```python
from build123d import *

# Parameters (mm, degrees)
SKETCH_W        = 30
SKETCH_H        = 200
PAD_DEPTH       = 10
POCKET_DEPTH    = 7.1
SKETCH002_W     = 200
SKETCH002_H     = 4.1
POCKET001_DEPTH = 7.1
SKETCH003_R     = 1.6
POCKET002_DEPTH = 25
SKETCH004_W     = 2.6
SKETCH004_H     = 5.7
POCKET003_DEPTH = 6.15
SKETCH006_W     = 200
SKETCH006_H     = 3
POCKET005_DEPTH = 5.9
POCKET006_DEPTH = 10
SKETCH008_W     = 5.9
SKETCH008_H     = 200
POCKET007_DEPTH = 3
POCKET008_DEPTH = 5.1
SKETCH010_W     = 30
SKETCH010_H     = 6.1
POCKET009_DEPTH = 5.1
POCKET010_DEPTH = 5


with BuildPart() as part:
    # Sketch → Pad (new body)
    with BuildSketch(Plane.XY):
        with Locations((15, 100)):
            Rectangle(SKETCH_W, SKETCH_H)
    extrude(amount=PAD_DEPTH)

    # Sketch001 (on Face4 of Pad) → Pocket (cut)
    with BuildSketch(Plane(origin=(0, 0, 0), x_dir=(0, -1, 0), z_dir=(-1, 0, 0))):
        Polygon((-199.7, 5.9), (-199.9, 0), (-179.9, 0), (-182.4, 5.9), align=None)
        Polygon((-167.6, 5.9), (-170.1, 0), (-154.9, 0), (-157.4, 5.9), align=None)
        Polygon((-142.6, 5.9), (-145.1, 0), (-129.9, 0), (-132.4, 5.9), align=None)
        Polygon((-117.6, 5.9), (-120.1, 0), (-104.9, 0), (-107.4, 5.9), align=None)
        Polygon((-92.6, 5.9), (-95.1, 0), (-79.9, 0), (-82.4, 5.9), align=None)
        Polygon((-67.6, 5.9), (-70.1, 0), (-54.9, 0), (-57.4, 5.9), align=None)
        Polygon((-42.6, 5.9), (-45.1, 0), (-29.9, 0), (-32.4, 5.9), align=None)
        Polygon((-17.6, 5.9), (-20.1, 0), (-4.9, 0), (-7.4, 5.9), align=None)
    extrude(amount=-POCKET_DEPTH, mode=Mode.SUBTRACT)

    # Sketch002 (on Face2 of Pocket) → Pocket001 (cut)
    with BuildSketch(Plane(origin=(0, 0, 0), x_dir=(0, -1, 0), z_dir=(-1, 0, 0))):
        with Locations((-100, 7.95)):
            Rectangle(SKETCH002_W, SKETCH002_H)
    extrude(amount=-POCKET001_DEPTH, mode=Mode.SUBTRACT)

    # Sketch003 (on Face9 of Pocket001) → Pocket002 (cut)
    with BuildSketch(Plane(origin=(7.1, 0, 0), x_dir=(0, -1, 0), z_dir=(-1, 0, 0))):
        with Locations((-37.5, 3)):
            Circle(SKETCH003_R)
        with Locations((-12.5, 3)):
            Circle(SKETCH003_R)
        with Locations((-62.5, 3)):
            Circle(SKETCH003_R)
        with Locations((-87.5, 3)):
            Circle(SKETCH003_R)
        with Locations((-112.5, 3)):
            Circle(SKETCH003_R)
        with Locations((-137.5, 3)):
            Circle(SKETCH003_R)
        with Locations((-162.5, 3)):
            Circle(SKETCH003_R)
        with Locations((-187.5, 3)):
            Circle(SKETCH003_R)
    extrude(amount=-POCKET002_DEPTH, mode=Mode.SUBTRACT)

    # Sketch004 (on Face2 of Pocket002) → Pocket003 (cut)
    with BuildSketch(Plane(origin=(0, 0, 0), x_dir=(1, 0, 0), z_dir=(0, 0, -1))):
        with Locations((15, -12.5)):
            Rectangle(SKETCH004_W, SKETCH004_H)
        with Locations((15, -37.5)):
            Rectangle(SKETCH004_W, SKETCH004_H)
        with Locations((15, -62.5)):
            Rectangle(SKETCH004_W, SKETCH004_H)
        with Locations((15, -87.5)):
            Rectangle(SKETCH004_W, SKETCH004_H)
        with Locations((15, -112.5)):
            Rectangle(SKETCH004_W, SKETCH004_H)
        with Locations((15, -137.5)):
            Rectangle(SKETCH004_W, SKETCH004_H)
        with Locations((15, -162.5)):
            Rectangle(SKETCH004_W, SKETCH004_H)
        with Locations((15, -187.5)):
            Rectangle(SKETCH004_W, SKETCH004_H)
    extrude(amount=-POCKET003_DEPTH, mode=Mode.SUBTRACT)

    # Sketch006 → Pocket005 (cut)
    with BuildSketch(Plane(origin=(0, 4.15414, -1.760229), x_dir=(-1, 0, 0), z_dir=(0, 0.920752, -0.390149))):
        with Locations((100, 8.5)):
            Rectangle(SKETCH006_W, SKETCH006_H)
    extrude(amount=-POCKET005_DEPTH, mode=Mode.SUBTRACT)

    # Sketch007 (on Face4 of Pocket005) → Pocket006 (cut)
    with BuildSketch(Plane.XY.offset(10)):
        Polygon((24.1, 20.1), (24.1, 4.9), (30, 7.4), (30, 17.6), align=None)
        Polygon((24.1, 45.1), (24.1, 29.9), (30, 32.4), (30, 42.6), align=None)
        Polygon((24.1, 70.1), (24.1, 54.9), (30, 57.4), (30, 67.6), align=None)
        Polygon((24.1, 95.1), (24.1, 79.9), (30, 82.4), (30, 92.6), align=None)
        Polygon((24.1, 120.1), (24.1, 104.9), (30, 107.4), (30, 117.6), align=None)
        Polygon((24.1, 145.1), (24.1, 129.9), (30, 132.4), (30, 142.6), align=None)
        Polygon((24.1, 170.1), (24.1, 154.9), (30, 157.4), (30, 167.6), align=None)
        Polygon((24.1, 195.1), (24.1, 179.9), (30, 182.4), (30, 192.6), align=None)
    extrude(amount=-POCKET006_DEPTH, mode=Mode.SUBTRACT)

    # Sketch008 (on Face4 of Pocket006) → Pocket007 (cut)
    with BuildSketch(Plane.XY.offset(10)):
        with Locations((27.05, 100)):
            Rectangle(SKETCH008_W, SKETCH008_H)
    extrude(amount=-POCKET007_DEPTH, mode=Mode.SUBTRACT)

    # Sketch009 (on Face6 of Pocket007) → Pocket008 (cut)
    with BuildSketch(Plane.XY.offset(10)):
        Polygon((7.4, 6.1), (22.6, 6.1), (20.1, 0), (9.9, 0), align=None)
    extrude(amount=-POCKET008_DEPTH, mode=Mode.SUBTRACT)

    # Sketch010 (on Face2 of Pocket008) → Pocket009 (cut)
    with BuildSketch(Plane(origin=(0, 0, 0), x_dir=(1, 0, 0), z_dir=(0, 0, -1))):
        with Locations((15, -196.95)):
            Rectangle(SKETCH010_W, SKETCH010_H)
    extrude(amount=-POCKET009_DEPTH, mode=Mode.SUBTRACT)

    # Sketch011 (on Face6 of Pocket009) → Pocket010 (cut)
    with BuildSketch(Plane.XY.offset(10)):
        Polygon((7.6, 200), (10.1, 194.1), (0, 194.1), (0, 200), align=None)
        Polygon((22.4, 200), (19.9, 194.1), (23.9, 194.1), (23.9, 200), align=None)
    extrude(amount=-POCKET010_DEPTH, mode=Mode.SUBTRACT)


solid = part.part
```
Here's how the part is built. I have some questions about the finished solid (model axes, mm). A direction names the side the tool comes from. Round coordinates to 2 decimals unless told otherwise and drop trailing zeros. Loops run counter-clockwise (first coordinate to the right, second up) from the corner with the lowest first, then second, coordinate; pieces in that order, holes last. Notation, with made-up numbers: (-27, -30.5) -> (7, -30.5) arc R17 cw to (7, -14.5) -> close; hole circle Ø5 at (47, -33). An arc over 180 degrees is marked (long way). Answer as CSV lines item,"result". Start each with the question number.
1. Imagine slicing it at B-B on z = 3. State how many separate pieces and enclosed holes the cut face has, plus the area to 3 significant figures.
2. I need wall thicknesses on probe 1 along X at (y, z) = (135, 0.75); probe 2 along Z at (x, y) = (25.5, 23); probe 3 along X at (y, z) = (43, 4.75). Which ranges of each line are inside material? Lowest first, please. Write a range as from..to.
3. For faces 1 (the face through (27.009, 181.132, 3.549)), 2 (the face through (27, 175, 7)), 3 (the face through (13.7, 164, 2)), which set-ups out of +Z, -Z, +X, -X, +Y, -Y let a thin tool reach every point of the face, with its end or its side?
4. Imagine slicing it at A-A on y = 173. Write out the boundary of the cut face in (x, z), plus the area to 3 significant figures.
5. If we mould it in two halves opening along Z, with no side actions, what happens to faces 4 (the face through (13.7, 11, 2)), 5 (the face through (4, 25, 5.9)), 6 (the face through (20.15, 186.02, 2.39))? For each: pulls with the +Z half, pulls with the -Z half, needs draft (parallel to the pull), parting line crosses it, or undercut.
6. I'm going to push flat-ended pins straight in: P1, Ø1, axis at y = 42.5, z = 8.5, coming from the +X side; P2, Ø4.5, axis at y = 87.5, z = 3.5, coming from the -X side; P3, Ø1.8, axis at x = 26.5, y = 149.5, coming from the +Z side; P4, Ø1.9, axis at y = 137.5, z = 3, coming from the +X side. Where does each tip first touch, or does it pass through?
Solution:
1,separate pieces,"10"
1,enclosed holes,"0"
1,area,"4,010 mm²"
2,probe 1,"7.1..13.7, 16.3..24.1"
2,probe 2,"0..7"
2,probe 3,"7.1..24.1, 29.06..30"
3,face 1,"+Z, -Z"
3,face 2,"+Z, +X, +Y, -Y"
3,face 3,"-Z"
4,outline,"(0, 0) -> (30, 0) -> (30, 7) -> (24.1, 7) -> (24.1, 10) -> (7.1, 10) -> (7.1, 5.9) -> (0, 5.9) -> close"
4,area,"253 mm²"
5,face 4,"needs draft"
5,face 5,"pulls with the +Z half"
5,face 6,"undercut"
6,P1,"x = 24.1"
6,P2,"x = 7.1"
6,P3,"z = 7"
6,P4,"through"
